from build123d import *

# Parameters (mm, degrees)
CUT_EXTRUDE1_DEPTH = 6.5
CUT_EXTRUDE2_DEPTH = 3


with BuildPart() as part:
    # Sketch1 → Revolve1 (revolve)
    with BuildSketch(Plane.XY):
        Polygon((0, 0), (0, 21), (73.5, 21), (73.5, 24), (133.5, 24), (133.5, 21), (241.5, 21), (241.5, 19.5), (298.5, 19.5), (298.5, 0), align=None)
    revolve(axis=Axis((298.5, 0, 0), (-1, 0, 0)))

    # Sketch3 → Cut-Extrude1 (cut)
    with BuildSketch(Plane.XY.offset(19.5)):
        with BuildLine():
            Line((312.375, -3.375), (284.625, -3.375))
            ThreePointArc((284.625, -3.375), (281.25, 0), (284.625, 3.375))
            Line((284.625, 3.375), (312.375, 3.375))
            ThreePointArc((312.375, 3.375), (315.75, 0), (312.375, -3.375))
        make_face()
    extrude(amount=-CUT_EXTRUDE1_DEPTH, mode=Mode.SUBTRACT)

    # Sketch4 → Cut-Extrude2 (cut)
    with BuildSketch(Plane.XY.offset(24)):
        with BuildLine():
            Line((97.5, 8.25), (109.5, 8.25))
            ThreePointArc((109.5, 8.25), (117.75, 0), (109.5, -8.25))
            Line((109.5, -8.25), (97.5, -8.25))
            ThreePointArc((97.5, -8.25), (89.25, 0), (97.5, 8.25))
        make_face()
    extrude(amount=-CUT_EXTRUDE2_DEPTH, mode=Mode.SUBTRACT)


solid = part.part
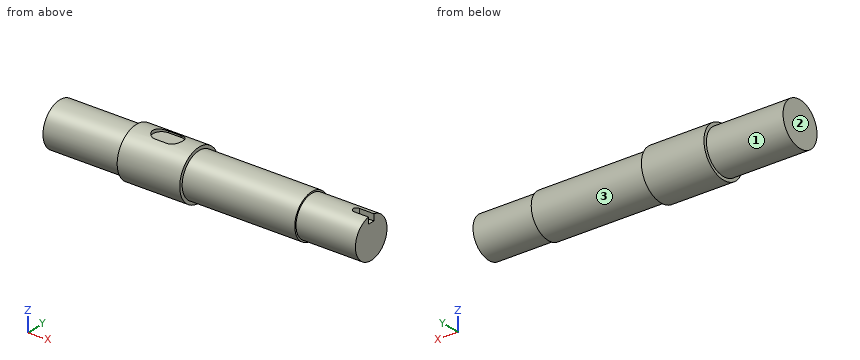
Source: CAD feature listing. Evaluate the final solid. Frame: model axes, mm. Face numbers are marked on the shaded views. A direction names the side the tool comes from. Give positions to 0.01 mm unless a question says otherwise; leave off trailing zeros. Write each loop counter-clockwise with the first axis right and the second up, starting at its lowest first coordinate (ties: lowest second). Pieces come first, ordered by that corner, then holes. Notation, with made-up numbers: M 61,0.25 L 84,0.25 A18 cw 84,22.25 Z; hole C -38.5,36.25 d3. An arc over 180 degrees is marked long. Return JSON: item names as keys, results as strings. Group by question number.
1) Cut plane C-C, the plane x = 277.5. Output: boundary loops of the cut face in (y, z), then the cut area to 3 significant figures.
2) Set-up query: the marked faces 1, 2 and 3. Return all of +Z, -Z, +X, -X, +Y, -Y with unobstructed straight access to the full face (end or side cutting, diameter ignored); none if empty.
3) Ray query, L1, parallel to Y at x = 276.5, z = 0.5; L2, parallel to Y at x = 168, z = -1.5; L3, parallel to X at y = 21.5, z = -6.5. Return the intervals inside material, ascending.
4) First-contact query: pin 1 Ø1.9 at (x, z) = (291.5, 15.5) entering from +Y; pin 2 Ø8 at (x, z) = (212.5, -2) entering from +Y; pin 3 Ø12 at (x, y) = (160.5, 11) entering from +Z. Flat tips, straight axial feed; report the tip coordinate or a pass-through.
5) Cut plane D-D, the plane z = -11.5. Output: boundary loops of the cut face in (x, y), then the cut area to 3 significant figures.
6) Cut plane B-B, the plane z = 0. Output: boundary loops of the cut face in (x, y).
7) Cut plane A-A, the plane y = 0. Output: boundary loops of the cut face in (x, z), then the cut area to 3 significant figures.
Data:
{
 "1": {"outline": "C 0,0 d39", "area": "1,190 mm²"},
 "2": {"face 1": "-X", "face 2": "+Z, -Z, -X, +Y, -Y", "face 3": "+X"},
 "3": {"L1": "y = -19.49 to 19.49", "L2": "y = -20.95 to 20.95", "L3": "x = 73.5 to 133.5"},
 "4": {"pin 1": "stops at y = 12.98", "pin 2": "stops at y = 21", "pin 3": "stops at z = 20.4"},
 "5": {"outline": "M 0,-17.57 L 73.5,-17.57 L 73.5,-21.07 L 133.5,-21.07 L 133.5,-17.57 L 241.5,-17.57 L 241.5,-15.75 L 298.5,-15.75 L 298.5,15.75 L 241.5,15.75 L 241.5,17.57 L 133.5,17.57 L 133.5,21.07 L 73.5,21.07 L 73.5,17.57 L 0,17.57 Z", "area": "10,700 mm²"},
 "6": {"outline": "M 0,-21 L 73.5,-21 L 73.5,-24 L 133.5,-24 L 133.5,-21 L 241.5,-21 L 241.5,-19.5 L 298.5,-19.5 L 298.5,19.5 L 241.5,19.5 L 241.5,21 L 133.5,21 L 133.5,24 L 73.5,24 L 73.5,21 L 0,21 Z"},
 "7": {"outline": "M 0,-21 L 73.5,-21 L 73.5,-24 L 133.5,-24 L 133.5,-21 L 241.5,-21 L 241.5,-19.5 L 298.5,-19.5 L 298.5,13 L 281.25,13 L 281.25,19.5 L 241.5,19.5 L 241.5,21 L 133.5,21 L 133.5,24 L 117.75,24 L 117.75,21 L 89.25,21 L 89.25,24 L 73.5,24 L 73.5,21 L 0,21 Z", "area": "12,500 mm²"}
}
